Can you work these out from the model? Positions are in its coordinate system, mm. A direction names the side the tool comes from. Give positions to 0.01 mm unless a question says otherwise; leave off trailing zeros. Loops run counter-clockwise (first coordinate to the right, second up) from the corner with the lowest first, then second, coordinate; pieces in that order, holes last. Notation, with made-up numbers: (18.25, 84) -> (68.25, 84) arc R11 ccw to (68.25, 89) -> close; hole circle Ø10 at (8.25, 61). An arc over 180 degrees is marked (long way). One line per question, with ' | ' between items.
from build123d import *

# Parameters (mm, degrees)
F0_W     = 7.82
F0_H     = 15.8
F0_R     = 2.43
F1_DEPTH = 9.58
F2_DEPTH = 10.98
F4_DEPTH = 8.28


with BuildPart() as f1:
    # F0 (on Top) → F1 (new body)
    with BuildSketch(Plane.XY):
        Rectangle(F0_W, F0_H)
        with Locations((0, -4.11)):
            Circle(F0_R, mode=Mode.SUBTRACT)
        with Locations((0, 4.1)):
            Circle(F0_R, mode=Mode.SUBTRACT)
        with Locations((0, -4.11)):
            Circle(F0_R)
        with Locations((0, 4.1)):
            Circle(F0_R)
    extrude(amount=F1_DEPTH)

    # F0 (on Top) → F2 (join)
    with BuildSketch(Plane.XY):
        with Locations((0, -4.11)):
            Circle(F0_R)
        with Locations((0, 4.1)):
            Circle(F0_R)
    extrude(amount=F2_DEPTH)

    # F3 (on face) → F4 (cut)
    with BuildSketch(Plane(origin=(0, 0, 0), x_dir=(1, 0, 0), z_dir=(0, 0, -1))):
        with BuildLine():
            Line((-2.43, -0.317888), (-2.43, -6.22))
            Line((-2.43, -6.22), (2.43, -6.22))
            Line((2.43, -6.22), (2.43, -0.606731))
            Line((2.43, -0.606731), (1.088562, -0.606731))
            ThreePointArc((1.088562, -0.606731), (-0.155715, -1.236463), (-1.205005, -0.317888))
            Line((-1.205005, -0.317888), (-2.43, -0.317888))
        make_face()
        with BuildLine():
            Line((-2.43, 6.22), (-2.43, 0.742112))
            Line((-2.43, 0.742112), (-1.001179, 0.742112))
            ThreePointArc((-1.001179, 0.742112), (0.165026, 1.235255), (1.160877, 0.453269))
            Line((1.160877, 0.453269), (2.43, 0.453269))
            Line((2.43, 0.453269), (2.43, 6.22))
            Line((2.43, 6.22), (-2.43, 6.22))
        make_face()
    extrude(amount=-F4_DEPTH, mode=Mode.SUBTRACT)


solid = f1.part
Q1. If I drill on probe 1 along Y at (x, z) = (1.25, 8); probe 2 along Y at (x, z) = (-2, 1.25); probe 3 along X at (y, z) = (-5.75, 6.25), over which ranges is the centre line in solid material (lowest first)? Write a range as from..to.
Entries:
probe 1: -7.9..-6.22, -0.45..0.61, 6.22..7.9 | probe 2: -7.9..-6.22, -0.74..0.32, 6.22..7.9 | probe 3: -3.91..-2.43, 2.43..3.91
Q2. On a 3-axis mill with a long thin cutter (end or side, diameter ignored), from which of +Z, -Z, +X, -X, +Y, -Y can I reach the whole of each face in a straight line? I mean faces 1 (the face through (2, 0.607, 4)), 2 (the face through (0, 4, 10.98)), 3 (the face through (-0.53, 1.73, 10.27)). Say none if no direction works.
Entries:
face 1: -Z | face 2: +Z, +X, -X, +Y, -Y | face 3: +Z
Q3. If we mould it in two halves opening along X, with no side actions, what happens to faces 4 (the face through (-0.3, -1.7, 10.3)), 5 (the face through (-3.91, 0, 5)), 6 (the face through (0, 0, 0)), 7 (the face through (2.43, 3, 4))? For each: pulls with the +X half, pulls with the -X half, needs draft (parallel to the pull), parting line crosses it, or undercut.
Entries:
face 4: parting line crosses it | face 5: pulls with the -X half | face 6: needs draft | face 7: undercut
Q4. If we section it at C-C (z = 5.5): Write out the boundary of the cut face in (x, y) (3 decimals), plus the area to 3 significant figures.
Entries:
outline: (-3.91, -7.9) -> (3.91, -7.9) -> (3.91, 7.9) -> (-3.91, 7.9) -> close; hole (-2.43, -6.22) -> (2.43, -6.22) -> (2.43, -0.453) -> (1.161, -0.453) arc R1.246 cw to (-1.001, -0.742) -> (-2.43, -0.742) -> close; hole (-2.43, 0.318) -> (-1.205, 0.318) arc R1.246 cw to (1.089, 0.607) -> (2.43, 0.607) -> (2.43, 6.22) -> (-2.43, 6.22) -> close | area: 70.6 mm²
Q5. If we section it at B-B (y = -4.11): Write out the boundary of the cut face in (x, z), plus the area to 3 significant figures.
Entries:
outline: (-3.91, 0) -> (-2.43, 0) -> (-2.43, 8.28) -> (2.43, 8.28) -> (2.43, 0) -> (3.91, 0) -> (3.91, 9.58) -> (2.43, 9.58) -> (2.43, 10.98) -> (-2.43, 10.98) -> (-2.43, 9.58) -> (-3.91, 9.58) -> close | area: 41.5 mm²
Q6. If we section it at A-A (x = 0): Write out the boundary of the cut face in (y, z).
Entries:
outline: (-7.9, 0) -> (-6.22, 0) -> (-6.22, 8.28) -> (-1.25, 8.28) -> (-1.25, 0) -> (1.25, 0) -> (1.25, 8.28) -> (6.22, 8.28) -> (6.22, 0) -> (7.9, 0) -> (7.9, 9.58) -> (6.53, 9.58) -> (6.53, 10.98) -> (1.67, 10.98) -> (1.67, 9.58) -> (-1.68, 9.58) -> (-1.68, 10.98) -> (-6.54, 10.98) -> (-6.54, 9.58) -> (-7.9, 9.58) -> close
Q7. For pin 1 Ø2 at (x, y) = (-3, 4.5) entering from -Z; pin 2 Ø1.5 at (x, y) = (-0.5, 3.5) entering from -Z, each with a flat end and sliding along its axis, tell me the tip position at first contact or that it passes through.
Entries:
pin 1: z = 0 | pin 2: z = 8.28
Q8. If we section it at D-D (x = 3.25): Write out the boundary of the cut face in (y, z), plus the area to 3 significant figures.
Entries:
outline: (-7.9, 0) -> (7.9, 0) -> (7.9, 9.58) -> (-7.9, 9.58) -> close | area: 151 mm²
